Part model, mm, in its own coordinate system. Give positions to 0.01 mm unless a question says otherwise; leave off trailing zeros. Write each loop counter-clockwise with the first axis right and the second up, starting at its lowest first coordinate (ties: lowest second). Pieces come first, ordered by that corner, then holes.
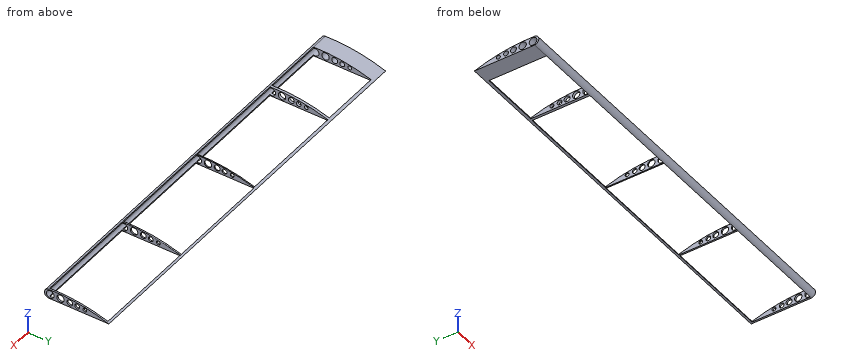
```python
from build123d import *

# Parameters (mm, degrees)
F1_DEPTH  = 290.83
F2_R      = 2.75814
F3_DEPTH  = 488.95
F4_R      = 2.656401
F5_DEPTH  = 389.89
F6_R      = 2.130296
F7_DEPTH  = 366.268
F8_R      = 1.744402
F9_DEPTH  = 536.702
F10_R     = 1.383816
F11_DEPTH = 596.646
F13_W     = 76.048613
F13_H     = 42.006582
F14_DEPTH = 226.06
F15_W     = 76.562449
F15_H     = 42.006582
F16_DEPTH = 224.028
F17_W     = 77.076297
F17_H     = 41.74966
F18_DEPTH = 220.98
F19_W     = 43.933488
F19_H     = 41.492738
F20_DEPTH = 92.71


with BuildPart() as f1:
    # F0 (on Right) → F1 (new body)
    with BuildSketch(Plane.YZ):
        with BuildLine():
            ThreePointArc((43.487221, 0), (22.067204, 5.454355), (0, 6.721488))
            ThreePointArc((0, 6.721488), (-3.002391, 3.360744), (0, 0))
            Line((0, 0), (43.487221, 0))
        make_face()
    extrude(amount=F1_DEPTH)

    # F2 (on Right) → F3 (cut)
    with BuildSketch(Plane.YZ):
        with Locations((1.214727, 3.320253)):
            Circle(F2_R)
    extrude(amount=F3_DEPTH, mode=Mode.SUBTRACT)

    # F4 (on Right) → F5 (cut)
    with BuildSketch(Plane.YZ):
        with Locations((8.665053, 3.482217)):
            Circle(F4_R)
    extrude(amount=F5_DEPTH, mode=Mode.SUBTRACT)

    # F6 (on Right) → F7 (cut)
    with BuildSketch(Plane.YZ):
        with Locations((15.305555, 3.320253)):
            Circle(F6_R)
    extrude(amount=F7_DEPTH, mode=Mode.SUBTRACT)

    # F8 (on Right) → F9 (cut)
    with BuildSketch(Plane.YZ):
        with Locations((20.650355, 2.996326)):
            Circle(F8_R)
    extrude(amount=F9_DEPTH, mode=Mode.SUBTRACT)

    # F10 (on Right) → F11 (cut)
    with BuildSketch(Plane.YZ):
        with Locations((26.157115, 2.672399)):
            Circle(F10_R)
    extrude(amount=F11_DEPTH, mode=Mode.SUBTRACT)

    # F13 (on offset) → F14 (cut)
    with BuildSketch(Plane.XY.offset(-41.656)):
        with Locations((251.576125, 21.003291)):
            Rectangle(F13_W, F13_H)
    extrude(amount=F14_DEPTH, mode=Mode.SUBTRACT)

    # F15 (on offset) → F16 (cut)
    with BuildSketch(Plane.XY.offset(-41.656)):
        with Locations((174.242907, 21.003291)):
            Rectangle(F15_W, F15_H)
    extrude(amount=F16_DEPTH, mode=Mode.SUBTRACT)

    # F17 (on offset) → F18 (cut)
    with BuildSketch(Plane.XY.offset(-41.656)):
        with Locations((96.652771, 20.87483)):
            Rectangle(F17_W, F17_H)
    extrude(amount=F18_DEPTH, mode=Mode.SUBTRACT)

    # F19 (on offset) → F20 (cut)
    with BuildSketch(Plane.XY.offset(-41.656)):
        with Locations((34.349431, 20.746369)):
            Rectangle(F19_W, F19_H)
    extrude(amount=F20_DEPTH, mode=Mode.SUBTRACT)


solid = f1.part
```
1) Saw through at A-A, the plane x = 261.5. Write the cut outline in (y, z), then the cut area to 3 significant figures.
Answers follow:
outline: (0, 0) - (0, 0.84) arc R2.76 cw to (0, 5.8) - (0, 6.72) arc R3.38 ccw to start; (42.01, 0) - (43.49, 0) arc R115.31 ccw to (42.01, 0.52) - close
area: 10.3 mm2
2) Saw through at B-B, the plane y = 31.5. Write the cut outline in (x, z), then the cut area to 3 significant figures.
Answers follow:
outline: (0, 0) - (12.38, 0) - (12.38, 3.59) - (0, 3.59) - close; (56.32, 0) - (58.11, 0) - (58.11, 3.59) - (56.32, 3.59) - close; (135.19, 0) - (135.96, 0) - (135.96, 3.59) - (135.19, 3.59) - close; (212.52, 0) - (213.55, 0) - (213.55, 3.59) - (212.52, 3.59) - close; (289.6, 0) - (290.83, 0) - (290.83, 3.59) - (289.6, 3.59) - close
area: 61.8 mm2
3) Wall check: L1, parallel to X at y = 4, z = 6.5; L2, parallel to Y at x = 209.5, z = 3.75; L3, parallel to Y at x = 117, z = 2.75. Give the ranges that are in metal, low to high.
Answers follow:
L1: x = 0 to 12.38, 56.32 to 58.11, 135.19 to 135.96, 212.52 to 213.55, 289.6 to 290.83
L2: y = -2.98 to -1.51
L3: y = -2.95 to -1.48
4) Pin check, flat tips, straight feed: pin 1 Ø4 at (y, z) = (20.5, 3.5) entering from +X; pin 2 Ø0.7 at (x, z) = (81, 6.5) entering from +Y; pin 3 Ø2 at (x, z) = (157, 1.5) entering from -Y. Stop position of each tip, or through.
Answers follow:
pin 1: stops at x = 290.83
pin 2: stops at y = 0
pin 3: stops at y = -2.89
